Verification items for the finished model (mm, model axes). A direction names the side the tool comes from. Coordinates: 2 decimals unless noted, no trailing zeros. Order: outer loops, then holes, each group sorted by start corner. A loop starts at its lowest first (then second) coordinate and runs counter-clockwise, first axis right, second up. Notation, with made-up numbers: (7, -14) -> (58, -14) arc R16 cw to (58, -5) -> close; hole circle Ø11 at (-29.5, 64). An arc over 180 degrees is marked (long way). Write each question's results on one line, items separated by ' | '. Start each with the question number.
(1) Cross-section at A-A on z = -5. Enter the section's corners in (x, y), and give its area (3 significant figures).
(2) Thickness scan on probe 1 along Z at (x, y) = (-7, 0.5); probe 2 along X at (y, z) = (0.5, -7); probe 3 along X at (y, z) = (1.7, 7). Record the ranges inside material, lowest first. Write a range as [from, to].
(3) Go/stop test with flat-tipped pins: pin 1 (0.5 mm diameter, centred on x = -1.5, y = 2.5, fed in from +Z); pin 2 (2.5 mm diameter, centred on x = -7, z = -7, fed in from +Y); pin 3 (1 mm diameter, centred on x = 6, z = -6, fed in from +Y). Record where each tip stops, or that it passes through.
(4) Cross-section at B-B on y = 0.85. Give the number of separate pieces and of enclosed holes in the cut face, and give its area (3 significant figures).
(5) Cross-section at D-D on z = 0.75. Enter the section's corners in (x, y), and give its area (3 significant figures).
(6) Set-up check for faces 1 (the flat face through (1, 2, -5.38)), 2 (the flat face through (-4.25, 2, 6)), 3 (the flat face through (-1.25, 2, 6)), 4 (the flat face through (1.1, 2, 7)): record each of +Z, -Z, +X, -X, +Y, -Y from which the full face is reachable in a straight line by a thin tool's end or side.
(7) Cross-section at C-C on x = -3.75. Enter the section's corners in (y, z), and give its area (3 significant figures).
(8) Draft check along Z on faces 5 (the flat face through (-2, 2, 2)), 6 (the flat face through (0.461, 2, 3)), 7 (the cylindrical face through (8.998, 0.818, -9.037)). Enter one of: +Z half, -Z half, draft (parallel to the pull), parting line (faces both ways), or undercut.
```python
from build123d import *

# Parameters (mm, degrees)
BOSS_EXTRU_1_DEPTH              = 1.66
DIAM_TRE_DU_PER_AGE_2_0_2_1_D   = 2
ESQUISSE4_R                     = 1.75
ENL_V_MAT_EXTRU_1_DEPTH         = 0.01
DIAM_TRE_DU_PER_AGE_0_8_0_8_1_D = 0.8
ESQUISSE7_W                     = 4
ESQUISSE7_H                     = 4
BOSS_EXTRU_2_DEPTH              = 1.6
ESQUISSE8_W                     = 3
ESQUISSE8_H                     = 1.7
BOSS_EXTRU_3_DEPTH              = 1.2
ESQUISSE9_W                     = 1.35
ESQUISSE9_H                     = 2.2
BOSS_EXTRU_4_DEPTH              = 1.2
ESQUISSE10_W                    = 1.35
ESQUISSE10_H                    = 1.35
ENL_V_MAT_EXTRU_2_DEPTH         = 0.01
ESQUISSE13_W                    = 1.35
ESQUISSE13_H                    = 2.2
BOSS_EXTRU_6_DEPTH              = 1.2
ESQUISSE15_W                    = 1.35
ESQUISSE15_H                    = 1.35
ENL_V_MAT_EXTRU_3_DEPTH         = 0.01
ESQUISSE18_W                    = 1.35
ESQUISSE18_H                    = 2.2
BOSS_EXTRU_7_DEPTH              = 1.2
ESQUISSE20_W                    = 1.35
ESQUISSE20_H                    = 1.35
ENL_V_MAT_EXTRU_5_DEPTH         = 0.01
ESQUISSE23_W                    = 1.35
ESQUISSE23_H                    = 2.2
BOSS_EXTRU_9_DEPTH              = 1.2
ESQUISSE25_W                    = 1.35
ESQUISSE25_H                    = 1.35
ENL_V_MAT_EXTRU_6_DEPTH         = 0.01
ESQUISSE27_W                    = 1.35
ESQUISSE27_H                    = 2.2
BOSS_EXTRU_10_DEPTH             = 1.2
ESQUISSE29_W                    = 1.35
ESQUISSE29_H                    = 1.35
ENL_V_MAT_EXTRU_7_DEPTH         = 0.01


with BuildPart() as part:
    # Esquisse1 → Boss.-Extru.1 (new body)
    with BuildSketch(Plane(origin=(0, 0, 0), x_dir=(1, 0, 0), z_dir=(0, 1, 0))):
        with BuildLine():
            Line((-7.25, 9.75), (7.25, 9.75))
            ThreePointArc((7.25, 9.75), (9.017766953, 9.017766953), (9.75, 7.25))
            Line((9.75, 7.25), (9.75, -7.25))
            ThreePointArc((9.75, -7.25), (9.017766953, -9.017766953), (7.25, -9.75))
            Line((7.25, -9.75), (-7.25, -9.75))
            ThreePointArc((-7.25, -9.75), (-9.017766953, -9.017766953), (-9.75, -7.25))
            Line((-9.75, -7.25), (-9.75, 7.25))
            ThreePointArc((-9.75, 7.25), (-9.017766953, 9.017766953), (-7.25, 9.75))
        make_face()
    extrude(amount=BOSS_EXTRU_1_DEPTH)

    # Diam_tre du per_age _2.0 _2_1 (through all)
    with Locations(Plane(origin=(0, 1.66, 0), x_dir=(1, 0, 0), z_dir=(0, 1, 0))):
        with Locations((-7, -7), (-7, 7)):
            Hole(DIAM_TRE_DU_PER_AGE_2_0_2_1_D / 2)

    # Esquisse4 → Enl_v. mat.-Extru.1 (cut)
    with BuildSketch(Plane(origin=(0, 1.66, 0), x_dir=(1, 0, 0), z_dir=(0, 1, 0))):
        with Locations(Location((-7, 7, 0), (0, 0, 270))):
            Circle(ESQUISSE4_R)
        with Locations(Location((-7, -7, 0), (0, 0, 270))):
            Circle(ESQUISSE4_R)
    extrude(amount=-ENL_V_MAT_EXTRU_1_DEPTH, mode=Mode.SUBTRACT)

    # Diam_tre du per_age _0.8 _0.8_1 (through all)
    with Locations(Plane(origin=(0, 1.66, 0), x_dir=(1, 0, 0), z_dir=(0, 1, 0))):
        with Locations((7.25, 7.5), (7.25, 5), (7.25, 2.5), (7.25, 0), (7.25, -2.5), (7.25, -5), (7.25, -7.5)):
            Hole(DIAM_TRE_DU_PER_AGE_0_8_0_8_1_D / 2)

    # Esquisse7 → Boss.-Extru.2 (add)
    with BuildSketch(Plane(origin=(0, 1.66, 0), x_dir=(1, 0, 0), z_dir=(0, 1, 0))):
        with Locations((-2.25, 0)):
            Rectangle(ESQUISSE7_W, ESQUISSE7_H)
    extrude(amount=BOSS_EXTRU_2_DEPTH)

    # Esquisse8 → Boss.-Extru.3 (add)
    with BuildSketch(Plane(origin=(0, 1.66, 0), x_dir=(1, 0, 0), z_dir=(0, 1, 0))):
        with Locations((-2.75, -6.4)):
            Rectangle(ESQUISSE8_W, ESQUISSE8_H)
    extrude(amount=BOSS_EXTRU_3_DEPTH)

    # Esquisse9 → Boss.-Extru.4 (add)
    with BuildSketch(Plane(origin=(0, 1.66, 0), x_dir=(1, 0, 0), z_dir=(0, 1, 0))):
        with Locations((-1.713640357, 6.480344191)):
            Rectangle(ESQUISSE9_W, ESQUISSE9_H)
    extrude(amount=BOSS_EXTRU_4_DEPTH)

    # Esquisse10 → Enl_v. mat.-Extru.2 (cut)
    with BuildSketch(Plane(origin=(0, 2.86, 0), x_dir=(1, 0, 0), z_dir=(0, 1, 0))):
        with Locations((-1.713640357, 6.480344191)):
            Rectangle(ESQUISSE10_W, ESQUISSE10_H)
    extrude(amount=-ENL_V_MAT_EXTRU_2_DEPTH, mode=Mode.SUBTRACT)

    # Esquisse13 → Boss.-Extru.6 (add)
    with BuildSketch(Plane(origin=(5.041533198, 1.66, 0.171739912), x_dir=(1, 0, 0), z_dir=(0, 1, 0))):
        with Locations((-3.905173555, 6.652084103)):
            Rectangle(ESQUISSE13_W, ESQUISSE13_H)
    extrude(amount=BOSS_EXTRU_6_DEPTH)

    # Esquisse15 → Enl_v. mat.-Extru.3 (cut)
    with BuildSketch(Plane(origin=(5.041533198, 2.86, 0.171739912), x_dir=(1, 0, 0), z_dir=(0, 1, 0))):
        with Locations((-3.905173555, 6.652084103)):
            Rectangle(ESQUISSE15_W, ESQUISSE15_H)
    extrude(amount=-ENL_V_MAT_EXTRU_3_DEPTH, mode=Mode.SUBTRACT)

    # Esquisse18 → Boss.-Extru.7 (add)
    with BuildSketch(Plane(origin=(3.245250957, 1.66, 3.023332502), x_dir=(1, 0, 0), z_dir=(0, 1, 0))):
        with Locations((-2.108891314, 4.803676693)):
            Rectangle(ESQUISSE18_W, ESQUISSE18_H)
    extrude(amount=BOSS_EXTRU_7_DEPTH)

    # Esquisse20 → Enl_v. mat.-Extru.5 (cut)
    with BuildSketch(Plane(origin=(3.245250957, 2.86, 3.023332502), x_dir=(1, 0, 0), z_dir=(0, 1, 0))):
        with Locations((-2.108891314, 4.803676693)):
            Rectangle(ESQUISSE20_W, ESQUISSE20_H)
    extrude(amount=-ENL_V_MAT_EXTRU_5_DEPTH, mode=Mode.SUBTRACT)

    # Esquisse23 → Boss.-Extru.9 (add)
    with BuildSketch(Plane(origin=(5.945511171, 1.66, 6.874523991), x_dir=(1, 0, 0), z_dir=(0, 1, 0))):
        with Locations((-4.809151527, 3.954868182)):
            Rectangle(ESQUISSE23_W, ESQUISSE23_H)
    extrude(amount=BOSS_EXTRU_9_DEPTH)

    # Esquisse25 → Enl_v. mat.-Extru.6 (cut)
    with BuildSketch(Plane(origin=(5.945511171, 2.86, 6.874523991), x_dir=(1, 0, 0), z_dir=(0, 1, 0))):
        with Locations((-4.809151527, 3.954868182)):
            Rectangle(ESQUISSE25_W, ESQUISSE25_H)
    extrude(amount=-ENL_V_MAT_EXTRU_6_DEPTH, mode=Mode.SUBTRACT)

    # Esquisse27 → Boss.-Extru.10 (add)
    with BuildSketch(Plane(origin=(2.244432679, 1.66, 9.735089798), x_dir=(1, 0, 0), z_dir=(0, 1, 0))):
        with Locations((-1.819432679, 3.085089798)):
            Rectangle(ESQUISSE27_W, ESQUISSE27_H)
    extrude(amount=BOSS_EXTRU_10_DEPTH)

    # Esquisse29 → Enl_v. mat.-Extru.7 (cut)
    with BuildSketch(Plane(origin=(2.244432679, 2.86, 9.735089798), x_dir=(1, 0, 0), z_dir=(0, 1, 0))):
        with Locations((-1.819432679, 3.085089798)):
            Rectangle(ESQUISSE29_W, ESQUISSE29_H)
    extrude(amount=-ENL_V_MAT_EXTRU_7_DEPTH, mode=Mode.SUBTRACT)


solid = part.part
```
Results are:
1) outline: (-9.75, 0) -> (6.85, 0) -> (6.85, 1.66) -> (-9.75, 1.66) -> close; (7.65, 0) -> (9.75, 0) -> (9.75, 1.66) -> (7.65, 1.66) -> close | area: 31.0 mm2
2) probe 1: z = [-9.75, -8], [-6, 6], [8, 9.75] | probe 2: x = [-9.75, -8], [-6, 9.75] | probe 3: x = [-4.25, -1.25], [-0.25, 1.1]
3) pin 1: stops at z = 7.25 | pin 2: stops at y = 1.65 | pin 3: stops at y = 1.66
4) separate pieces: 1 | enclosed holes: 9 | area: 365 mm2
5) outline: (-9.75, 0) -> (9.75, 0) -> (9.75, 1.66) -> (-0.25, 1.66) -> (-0.25, 3.26) -> (-4.25, 3.26) -> (-4.25, 1.66) -> (-9.75, 1.66) -> close | area: 38.8 mm2
6) face 1: +X, -X, +Y | face 2: +Z, -Z, -X, +Y | face 3: +Z, +Y | face 4: +Z, +X, +Y
7) outline: (0, -9.75) -> (1.66, -9.75) -> (1.66, -2) -> (3.26, -2) -> (3.26, 2) -> (1.66, 2) -> (1.66, 5.55) -> (2.86, 5.55) -> (2.86, 7.25) -> (1.66, 7.25) -> (1.66, 9.75) -> (0, 9.75) -> close | area: 40.8 mm2
8) face 5: undercut | face 6: draft | face 7: -Z half
